Can you work these out from the model? Positions are in its coordinate system, mm. Coordinates: 2 decimals unless noted, no trailing zeros. Order: outer loops, then holes, each group sorted by start corner. A loop starts at its lowest first (then second) coordinate and runs counter-clockwise, first axis right, second up. Notation, with made-up numbers: (48, 63.25) - (91, 63.25) arc R33 cw to (91, 94.25) - close; hole circle Ø3 at (66.5, -24.5). An arc over 180 degrees is marked (long way). Return JSON: item names as keys, results as strings. Group by question number.
1) If I drill on line 1 along Z through (x, y) = (0.5, 2.25); line 2 along Z through (x, y) = (1, 2.75); line 3 along X through (y, z) = (5.5, -83.5), over which ranges is the centre line in solid material (lowest first)?
2) Imagine slicing it at B-B (z = -21). Write out the boundary of the cut face in (x, y), and give its area (3 significant figures).
3) Imagine slicing it at A-A (y = 1.75). Give the number of separate pieces and of enclosed holes in the cut face, and give its area (3 significant figures).
4) For pin 1 Ø1.5 at (y, z) = (2, 39.5) entering from -X; pin 2 Ø1.5 at (x, y) = (-48.5, 0.5) entering from -Z; pin 3 Ø4.5 at (x, z) = (0.05, -97.28) entering from -Y; pin 4 Ø1.5 at (y, z) = (5, 64.5) entering from -X, each with a flat end and sliding along its axis, tell me the tip position at first contact or that it passes through.
5) Imagine slicing it at C-C (x = -42.5). Write out the boundary of the cut face in (y, z), and give its area (3 significant figures).
6) If we mould it in two halves opening along Z, with no side actions, what happens to faces 1 (the face through (1, 0, -1)), 2 (the face through (-102.283, 3.131, -22.713)), 3 (the face through (-86.486, 3.219, -47.447)), 4 (the face through (94.808, 3.219, -0.083))? For each: pulls with the +Z half, pulls with the -Z half, needs draft (parallel to the pull), parting line crosses it, or undercut.
```python
from build123d import *

# Parameters (mm, degrees)
SKETCH2_R          = 104.775
FACE_PLATE_DEPTH   = 6.35
SKETCH3_R          = 2.5527
CUT_EXTRUDE1_DEPTH = 6.35
CIRPATTERN1_COUNT  = 12


with BuildPart() as part:
    # Sketch2 → Face Plate (new body)
    with BuildSketch(Plane(origin=(0, 0, 0), x_dir=(1, 0, 0), z_dir=(0, 1, 0))):
        with Locations(Location((0, 0, 0), (0, 0, 270))):
            Circle(SKETCH2_R)
    extrude(amount=FACE_PLATE_DEPTH)

    # Sketch3 → Cut-Extrude1 (cut)
    with BuildSketch(Plane(origin=(0, 6.35, 0), x_dir=(1, 0, 0), z_dir=(0, 1, 0))):
        with Locations(Location((-84.221187023, 48.625125, 0), (0, 0, 270))):
            Circle(SKETCH3_R)
    cut_extrude1 = extrude(amount=-CUT_EXTRUDE1_DEPTH, mode=Mode.SUBTRACT)

    # CirPattern1: Cut-Extrude1 ×12 about axis
    cirpattern1_axis = Axis((0.050022276, 0, 0.028880374), (0, 1, 0))
    for i in range(1, CIRPATTERN1_COUNT):
        add(cut_extrude1.rotate(cirpattern1_axis, i * 360 / CIRPATTERN1_COUNT), mode=Mode.SUBTRACT)


solid = part.part
```
Calculated:
{
 "1": {"line 1": "-104.77 to -99.79, -94.77 to 94.82, 99.85 to 104.77", "line 2": "-104.77 to -99.65, -94.91 to 94.97, 99.71 to 104.77", "line 3": "-63.29 to -51.05, -46.16 to 46.26, 51.15 to 63.29"},
 "2": {"outline": "(-102.65, 0) - (102.65, 0) - (102.65, 6.35) - (-102.65, 6.35) - close", "area": "1,300 mm2"},
 "3": {"separate pieces": "1", "enclosed holes": "12", "area": "34,200 mm2"},
 "4": {"pin 1": "x = -97.35", "pin 2": "z = -93.26", "pin 3": "through", "pin 4": "x = -83.15"},
 "5": {"outline": "(0, -95.77) - (6.35, -95.77) - (6.35, 95.77) - (0, 95.77) - close", "area": "1,220 mm2"},
 "6": {"face 1": "needs draft", "face 2": "parting line crosses it", "face 3": "undercut", "face 4": "undercut"}
}
